Drawing for the job (mm, zero at the part's lowest x, y, z). Coordinates: 2 decimals unless noted, no trailing zeros. Write each loop counter-clockwise with the first axis right and the second up, starting at its lowest first coordinate (ties: lowest second). Pieces come first, ordered by that corner, then holes. Notation, with made-up numbers: M -30.75,54 L -10.75,54 A24 cw -10.75,67 Z; hole C 46.25,-35 d6. An arc over 180 degrees is marked long. Use CSV: the item, a comma, the result in double quotes. Start each with the question number.
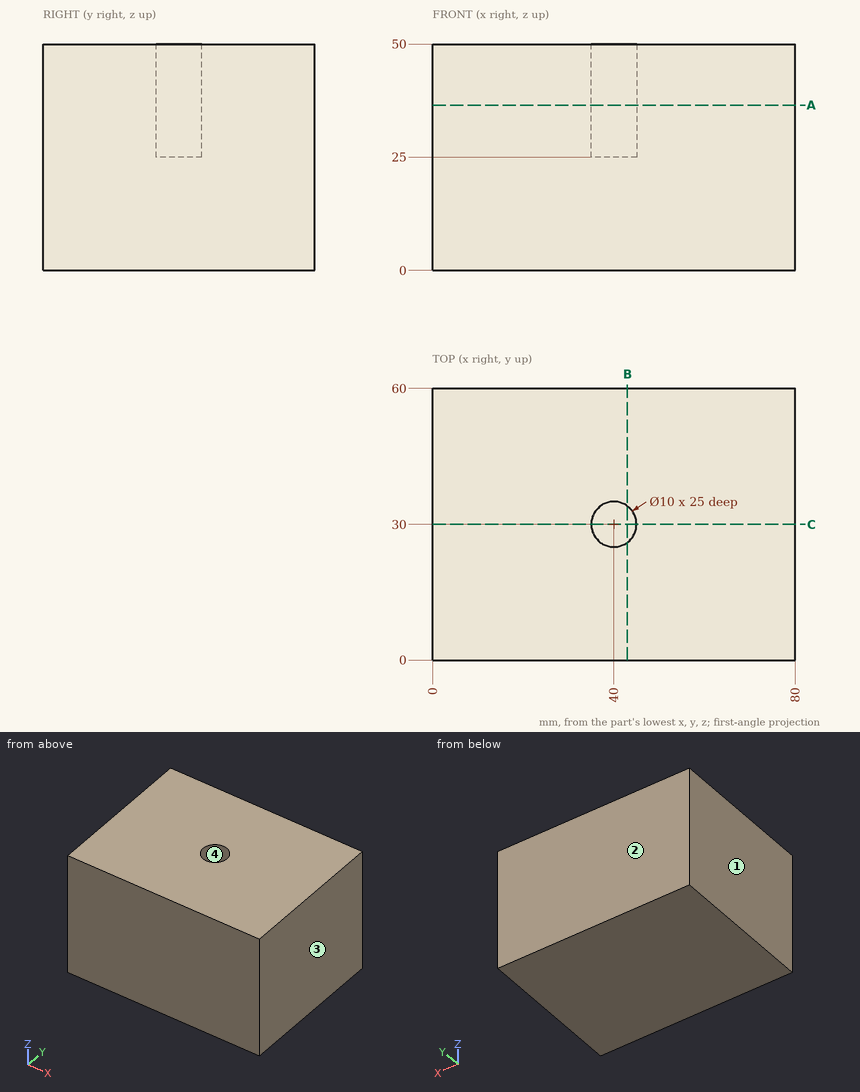
1) Drop a flat-ended pin along its axis: P1, Ø5, axis at x = 40, y = 32, coming from the +Z side. Give the stop position or say it passes through.
2) Two-plate mould, pull along X, no slides. Class the marked faces 1, 2, 3 and 4: pulls with the +X half, pulls with the -X half, needs draft (parallel to the pull), parting line crosses it, or undercut.
3) Band-saw the part on B-B on x = 43. List the corners of the cut face in (y, z), then the cut area to 3 significant figures.
4) Band-saw the part on A-A on z = 36.5. List the corners of the cut face in (x, y), then the cut area to 3 significant figures.
5) Band-saw the part on C-C on y = 30. List the corners of the cut face in (x, z).
6) Wall check: L1, parallel to Y at x = 40, z = 42; L2, parallel to Y at x = 43, z = 44.5. Give the ranges that are in metal, low to high. Write a range as [from, to].
Findings below:
1,P1,"stops at z = 25"
2,face 1,"pulls with the -X half"
2,face 2,"needs draft"
2,face 3,"pulls with the +X half"
2,face 4,"undercut"
3,outline,"M 0,0 L 60,0 L 60,50 L 34,50 L 34,25 L 26,25 L 26,50 L 0,50 Z"
3,area,"2,800 mm2"
4,outline,"M 0,0 L 80,0 L 80,60 L 0,60 Z; hole C 40,30 d10"
4,area,"4,720 mm2"
5,outline,"M 0,0 L 80,0 L 80,50 L 45,50 L 45,25 L 35,25 L 35,50 L 0,50 Z"
6,L1,"y = [0, 25], [35, 60]"
6,L2,"y = [0, 26], [34, 60]"
